```python
from build123d import *

# Parameters (mm, degrees)
F0_W     = 60
F0_H     = 60
F1_DEPTH = 20
F2_W     = 60
F2_H     = 5
F3_DEPTH = 8
F4_R     = 5
F5_DEPTH = 15
F6_SIZE  = 2


with BuildPart() as f1:
    # F0 (on Top) → F1 (new body)
    with BuildSketch(Plane.XY):
        Rectangle(F0_W, F0_H)
    extrude(amount=F1_DEPTH)

    # F2 (on face) → F3 (cut)
    with BuildSketch(Plane.XY.offset(20)):
        with Locations((0, 16.9222388044)):
            Rectangle(F2_W, F2_H)
    extrude(amount=-F3_DEPTH, mode=Mode.SUBTRACT)

    # F4 (on face) → F5 (cut)
    with BuildSketch(Plane.XY.offset(20)):
        with Locations((0, -20)):
            Circle(F4_R)
        with Locations((15, -20)):
            Circle(F4_R)
        with Locations((-15, -20)):
            Circle(F4_R)
    extrude(amount=-F5_DEPTH, mode=Mode.SUBTRACT)

    # F6
    f6_edges = [f1.edges().sort_by_distance(p)[0] for p in [
        (0, -30, 20),
        (30, -7.788881, 20),
        (30, 24.711119, 20),
        (0, 30, 20),
        (-30, -7.788881, 20),
        (-30, 24.711119, 20),
        (10, -20, 20),
        (-5, -20, 20),
        (-20, -20, 20),
        (0, 19.422239, 20),
        (0, 14.422239, 20),
        (30, -30, 10),
        (-30, -30, 10),
        (-30, 30, 10),
        (30, 30, 10),
    ]]
    chamfer(f6_edges, length=F6_SIZE)


solid = f1.part
```
Geometry check sheet. Reference: the model listing, model coordinates, mm. A direction names the side the tool comes from. Round coordinates to 2 decimals unless told otherwise and drop trailing zeros. Loops run counter-clockwise (first coordinate to the right, second up) from the corner with the lowest first, then second, coordinate; pieces in that order, holes last. Notation, with made-up numbers: (-23, 59.5) - (34, 59.5) arc R22 cw to (34, 85.5) - close; hole circle Ø9 at (-13, 72.5). An arc over 180 degrees is marked (long way). Write each question's results on one line, items separated by ' | '. Start each with the question number.
Q1. Cross-section at C-C on x = -15. Enter the section's corners in (y, z), and give its area (3 significant figures).
Q2. Gauge pin test, flat ends, axial feed: P1, Ø1.5, axis at x = -6.5, y = 18, coming from the +Z side; P2, Ø3, axis at x = 2.5, y = -18, coming from the +Z side. Record the tip position at first contact, or that the pin passes through.
Q3. Thickness scan on line 1 (X direction, y = -16.5, z = 5.5); line 2 (Z direction, x = 23, y = 13); line 3 (Y direction, x = 6, z = 15.25). Record the ranges inside material, lowest first. Write a range as [from, to].
Q4. Release check for a two-part mould opening along Y. For faces 4 (the flat face through (0, 30, 9)), 5 (the flat face through (29, 25, 19)), 6 (the flat face through (-0.42, 20.41, 18.99)) record: +Y half, -Y half, draft (parallel to the pull), parting line (faces both ways), or undercut.
Q5. Cross-section at B-B on z = 6.75. Enter the section's corners in (x, y), and give its area (3 significant figures).
Q6. Access from +Z, -Z, +X, -X, +Y, -Y to the whole of each face (thin tool, end or side, straight path). Record for faces 1 (the flat face through (29, -29, 9)), 2 (the flat face through (0, 14.422, 15)), 3 (the cylindrical face through (-16.08, -24.88, 11.59)).
Q7. Cross-section at A-A on z = 14.25. Enter the section's corners in (x, y), and give its area (3 significant figures).
Q8. Cross-section at D-D on y = -20. Enter the section's corners in (x, z).
Answers below:
1) outline: (-30, 0) - (30, 0) - (30, 18) - (28, 20) - (21.42, 20) - (19.42, 18) - (19.42, 12) - (14.42, 12) - (14.42, 18) - (12.42, 20) - (-13, 20) - (-15, 18) - (-15, 5) - (-25, 5) - (-25, 18) - (-27, 20) - (-28, 20) - (-30, 18) - close | area: 998 mm²
2) P1: stops at z = 12 | P2: stops at z = 5
3) line 1: x = [-30, -18.57], [-11.43, -3.57], [3.57, 11.43], [18.57, 30] | line 2: z = [0, 19.42] | line 3: y = [-30, 14.42], [19.42, 30]
4) face 4: +Y half | face 5: draft | face 6: undercut
5) outline: (-30, -28) - (-28, -30) - (28, -30) - (30, -28) - (30, 28) - (28, 30) - (-28, 30) - (-30, 28) - close; hole circle Ø10 at (-15, -20); hole circle Ø10 at (0, -20); hole circle Ø10 at (15, -20) | area: 3,360 mm²
6) face 1: +Z, -Z, +X, -Y | face 2: +Z, +X, -X | face 3: +Z
7) outline: (-30, -28) - (-28, -30) - (28, -30) - (30, -28) - (30, 14.42) - (-30, 14.42) - close; (-30, 19.42) - (30, 19.42) - (30, 28) - (28, 30) - (-28, 30) - (-30, 28) - close; hole circle Ø10 at (-15, -20); hole circle Ø10 at (0, -20); hole circle Ø10 at (15, -20) | area: 3,060 mm²
8) outline: (-30, 0) - (30, 0) - (30, 18) - (28, 20) - (22, 20) - (20, 18) - (20, 5) - (10, 5) - (10, 18) - (8, 20) - (7, 20) - (5, 18) - (5, 5) - (-5, 5) - (-5, 18) - (-7, 20) - (-8, 20) - (-10, 18) - (-10, 5) - (-20, 5) - (-20, 18) - (-22, 20) - (-28, 20) - (-30, 18) - close
